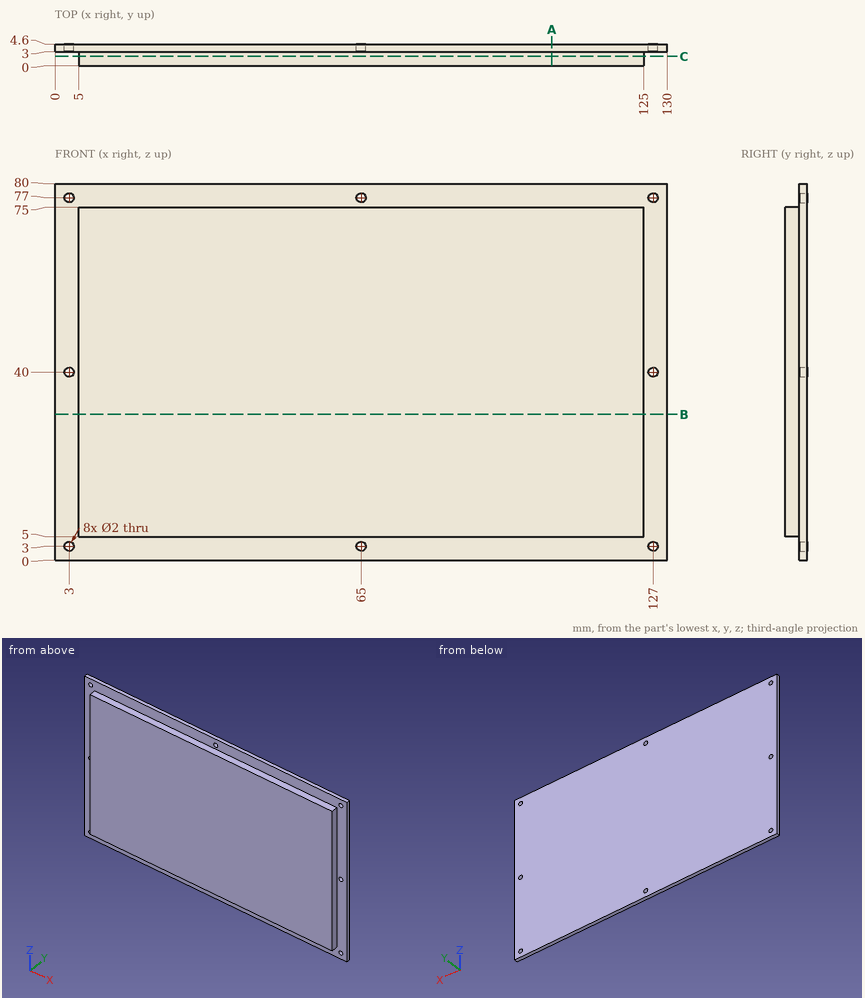
The drawing under review shows one solid part. Ordinate dimensions are in mm from its lowest x, y, z. Give positions to 0.01 mm unless a question says otherwise; leave off trailing zeros. Loops run counter-clockwise (first coordinate to the right, second up) from the corner with the lowest first, then second, coordinate; pieces in that order, holes last. Notation, with made-up numbers: M 29.5,14 L 41.5,14 A29 ccw 41.5,37 Z; hole C 54.25,89.25 d3. An arc over 180 degrees is marked long. One line per item, written item: value. Start each with the question number.
Q1. Add section C-C (y = 1.95). Give the boundary of the cut face in (x, z).
Q2. Add section A-A (x = 105.5). Give the boundary of the cut face in (y, z).
Q3. Clearance check with flat-ended pins moving along their axes: pin 1 Ø3 at (x, z) = (127, 3) entering from -Y; pin 2 Ø2.5 at (x, y) = (59, 1.5) entering from +Z; pin 3 Ø0.9 at (y, z) = (1.5, 55.5) entering from +X. State where each tip first meets the part, or that it passes through.
Q4. For L1, parallel to X at y = 3.75, z = 77; L2, parallel to Z at x = 3, y = 3.8; L3, parallel to Z at x = 65, y = 3.95, list the stretches that pass through material, from the lowest coordinate up.
Q5. Add section B-B (z = 31). Give the boundary of the cut face in (x, y).
Reply:
1. outline: M 5,5 L 125,5 L 125,75 L 5,75 Z
2. outline: M 0,5 L 3,5 L 3,0 L 4.6,0 L 4.6,80 L 3,80 L 3,75 L 0,75 Z
3. pin 1: y = 3
3. pin 2: z = 75
3. pin 3: x = 125
4. L1: 0 to 2, 4 to 64, 66 to 126, 128 to 130
4. L2: 0 to 2, 4 to 39, 41 to 76, 78 to 80
4. L3: 0 to 2, 4 to 76, 78 to 80
5. outline: M 0,3 L 5,3 L 5,0 L 125,0 L 125,3 L 130,3 L 130,4.6 L 0,4.6 Z
